```python
from build123d import *

# Parameters (mm, degrees)
SKETCH1_R           = 82.55
BOSS_EXTRUDE2_DEPTH = 6.35
SKETCH2_W           = 40.9
SKETCH2_H           = 20.6
CUT_EXTRUDE1_DEPTH  = 3.175
CUT_EXTRUDE2_REACH  = 118.916
SKETCH3_R           = 1.65
CIRPATTERN1_COUNT   = 4
BOSS_EXTRUDE3_START = 32.824999914
SKETCH5_R           = 4.825
SKETCH5_R_2         = 1.65
BOSS_EXTRUDE3_DEPTH = 32.824999914
CIRPATTERN3_COUNT   = 4
SKETCH4_R           = 2.9
CUT_EXTRUDE3_DEPTH  = 20
CIRPATTERN4_COUNT   = 4
BOSS_EXTRUDE5_DEPTH = 20
FILLET1_R           = 1.5


with BuildPart() as part:
    # Sketch1 → Boss-Extrude2 (new body)
    with BuildSketch(Plane(origin=(0, 0, 0), x_dir=(1, 0, 0), z_dir=(0, 1, 0))):
        with Locations(Location((0, 0, 0), (0, 0, 270))):
            Circle(SKETCH1_R)
    extrude(amount=BOSS_EXTRUDE2_DEPTH)

    # Sketch2 → Cut-Extrude1 (cut)
    with BuildSketch(Plane(origin=(0, 6.35, 0), x_dir=(1, 0, 0), z_dir=(0, 1, 0))):
        Rectangle(SKETCH2_W, SKETCH2_H)
    extrude(amount=-CUT_EXTRUDE1_DEPTH, mode=Mode.SUBTRACT)

    # Sketch3 → Cut-Extrude2 (cut, up to next)
    with BuildSketch(Plane(origin=(0, 6.35, 0), x_dir=(1, 0, 0), z_dir=(0, 1, 0)), mode=Mode.PRIVATE) as cut_extrude2_sk1:
        with Locations(Location((0, 76.2, 0), (0, 0, 270))):
            Circle(SKETCH3_R)
    cut_extrude2_tool1 = extrude(cut_extrude2_sk1.sketch, amount=-CUT_EXTRUDE2_REACH, mode=Mode.PRIVATE) & part.part
    cut_extrude2 = cut_extrude2_tool1.solids().sort_by_distance((0, 6.35, -76.2))[0]
    add(cut_extrude2, mode=Mode.SUBTRACT)

    # CirPattern1: Cut-Extrude2 ×4 about axis
    cirpattern1_axis = Axis((0, 0, 0), (0, 1, 0))
    for i in range(1, CIRPATTERN1_COUNT):
        add(cut_extrude2.rotate(cirpattern1_axis, i * 360 / CIRPATTERN1_COUNT), mode=Mode.SUBTRACT)

    # Sketch5 → Boss-Extrude3 (add)
    with BuildSketch(Plane(origin=(0, 6.35, 0), x_dir=(1, 0, 0), z_dir=(0, 1, 0)).offset(BOSS_EXTRUDE3_START)):
        with Locations(Location((0, 76.2, 0), (0, 0, 270))):
            Circle(SKETCH5_R)
        with Locations(Location((0, 76.2, 0), (0, 0, 270))):
            Circle(SKETCH5_R_2, mode=Mode.SUBTRACT)
    boss_extrude3 = extrude(amount=-BOSS_EXTRUDE3_DEPTH)

    # CirPattern3: Boss-Extrude3 ×4 about axis
    cirpattern3_axis = Axis((0, 0, 0), (0, 1, 0))
    for i in range(1, CIRPATTERN3_COUNT):
        add(boss_extrude3.rotate(cirpattern3_axis, i * 360 / CIRPATTERN3_COUNT))

    # Sketch4 → Cut-Extrude3 (cut)
    with BuildSketch(Plane.XZ):
        with Locations(Location((-76.2, 0, 0), (0, 0, 270))):
            Circle(SKETCH4_R)
    cut_extrude3 = extrude(amount=-CUT_EXTRUDE3_DEPTH, mode=Mode.SUBTRACT)

    # CirPattern4: Cut-Extrude3 ×4 about axis
    cirpattern4_axis = Axis((0, 0, 0), (0, 1, 0))
    for i in range(1, CIRPATTERN4_COUNT):
        add(cut_extrude3.rotate(cirpattern4_axis, i * 360 / CIRPATTERN4_COUNT), mode=Mode.SUBTRACT)

    # Sketch6 → Boss-Extrude5 (add)
    with BuildSketch(Plane(origin=(0, 6.35, 0), x_dir=(1, 0, 0), z_dir=(0, 1, 0))):
        Polygon((-20.45, 10.3), (20.45, 10.3), (20.45, 5), (23.45, 5), (23.45, 13.3), (-23.45, 13.3), (-23.45, -13.3), (23.45, -13.3), (23.45, -5), (20.45, -5), (20.45, -10.3), (-20.45, -10.3), align=None)
    extrude(amount=BOSS_EXTRUDE5_DEPTH)

    # Fillet1
    fillet1_edges = [part.edges().sort_by_distance(p)[0] for p in [
        (23.45, 26.35, -9.15),
        (0, 26.35, -13.3),
        (-23.45, 26.35, 0),
        (0, 26.35, 13.3),
        (23.45, 26.35, 9.15),
        (21.95, 26.35, 5),
        (20.45, 26.35, 7.65),
        (0, 26.35, 10.3),
        (-20.45, 26.35, 0),
        (0, 26.35, -10.3),
        (20.45, 26.35, -7.65),
        (21.95, 26.35, -5),
    ]]
    fillet(fillet1_edges, radius=FILLET1_R - 0.0001)  # a hair under: the kernel refuses the full size


solid = part.part
```
Geometry: final body of the model. Coordinates: model frame, mm. A direction names the side the tool comes from. Round coordinates to 2 decimals unless told otherwise and drop trailing zeros. Write each loop counter-clockwise with the first axis right and the second up, starting at its lowest first coordinate (ties: lowest second). Pieces come first, ordered by that corner, then holes.
Item 1: Pin query (flat end, axial travel): P1, Ø5.5, axis at x = -2, y = 15.5, coming from the +Z side (3 decimals); P2, Ø12, axis at x = -7.5, z = 1.5, coming from the +Y side (3 decimals); P3, Ø1.5, axis at x = 22, y = 17, coming from the -Z side; P4, Ø2, axis at x = 76.2, z = 0, coming from the +Y side. Return the tip coordinate at first contact, or that it passes through.
Item 2: Mould query, pull axis Z, two halves, no side actions, for faces 1 (the face through (0, 20, 78.1)), 2 (the face through (23.45, 15, -9)), 3 (the face through (-71.6, 22.99, -1.45)). Classes: +Z half, -Z half, draft (parallel to the pull), parting line (faces both ways), or undercut.
Item 3: Section query A-A (y = 31.5). Return loops of the section in (x, z) (3 decimals).
Item 4: Set-up query: faces 4 (the face through (73.325, 9.86, -0.378)), 5 (the face through (-23.45, 15, 0)), 6 (the face through (0, 39.175, -74)), 7 (the face through (81.848, 3.131, -10.746)), 8 (the face through (4.07, 22.99, -73.61)). Return all of +Z, -Z, +X, -X, +Y, -Y with unobstructed straight access to the full face (end or side cutting, diameter ignored); none if empty.
Item 5: Section query C-C (z = -41.5). Return loops of the section in (x, y).
Item 6: Material intervals for L1, parallel to Z at x = -76.2, y = 27.5 (3 decimals); L2, parallel to Z at x = 76.2, y = 7.25 (3 decimals); L3, parallel to Y at x = -41, z = -67.5, sorted ascending.
Completed:
1. P1: stops at z = 81.025
1. P2: stops at y = 3.175
1. P3: stops at z = -13.3
1. P4: passes through
2. face 1: undercut
2. face 2: draft
2. face 3: parting line
3. outline: circle Ø9.65 at (-76.2, 0); circle Ø9.65 at (0, -76.2); circle Ø9.65 at (0, 76.2); circle Ø9.65 at (76.2, 0); hole circle Ø3.3 at (-76.2, 0); hole circle Ø3.3 at (0, -76.2); hole circle Ø3.3 at (0, 76.2); hole circle Ø3.3 at (76.2, 0)
4. face 4: -Y
4. face 5: +Z, -Z, +Y
4. face 6: +Z, -Z, +X, -X, +Y
4. face 7: +Y, -Y
4. face 8: +Y
5. outline: (-71.36, 0) - (71.36, 0) - (71.36, 6.35) - (-71.36, 6.35) - close
6. L1: z = -4.825 to -1.65, 1.65 to 4.825
6. L2: z = -4.825 to -2.9, 2.9 to 4.825
6. L3: y = 0 to 6.35
